from build123d import *

# Parameters (mm, degrees)
F0_W     = 66.532835
F0_H     = 58.002986
F1_DEPTH = 25.4
F2_R     = 10


with BuildPart() as f1:
    # F0 (on Top) → F1 (new body)
    with BuildSketch(Plane.XY):
        with Locations((-3.070745, 4.776716)):
            Rectangle(F0_W, F0_H)
    extrude(amount=F1_DEPTH)

    # F2
    f2_edges = [f1.edges().sort_by_distance(p)[0] for p in [
        (-3.070746, 33.778209, 25.4),
    ]]
    fillet(f2_edges, radius=F2_R)


solid = f1.part
Read the model definition and answer for the solid it produces. Units are mm, in the model's axes. Round coordinates to 2 decimals unless told otherwise and drop trailing zeros. Order: outer loops, then holes, each group sorted by start corner. A loop starts at its lowest first (then second) coordinate and runs counter-clockwise, first axis right, second up.
1) A flat-ended cylindrical pin translates along its axis: pin 1 (1 mm diameter, centred on x = -1, z = 17.5, fed in from +Y). Find the tip coordinate at first contact, or state that the pin passes through.
2) Straight lines are drawn through the part: L1, parallel to Y at x = -28.5, z = 15.75; L2, parallel to Z at x = -19.5, y = 27; L3, parallel to Y at x = 1.5, z = 19. For each, find the intervals that lie inside material, in ascending order.
3) The part is cut by section B-B on z = 21.25. Write down the section's boundary in (x, y), plus the area to 3 significant figures.
4) The part is cut by section A-A on y = 28. Write down the section's boundary in (x, z), plus the area to 3 significant figures.
Resolved:
1. pin 1: stops at y = 33.65
2. L1: y = -24.22 to 33.77
2. L2: z = 0 to 24.87
2. L3: y = -24.22 to 33.11
3. outline: (-36.34, -24.22) - (30.2, -24.22) - (30.2, 31.89) - (-36.34, 31.89) - close
3. area: 3,730 mm2
4. outline: (-36.34, 0) - (30.2, 0) - (30.2, 24.47) - (-36.34, 24.47) - close
4. area: 1,630 mm2
